For this review, take the finished solid that the model builds, in its own axes (mm). A direction names the side the tool comes from. Give positions to 0.01 mm unless a question says otherwise; leave off trailing zeros. Order: outer loops, then holes, each group sorted by start corner. A loop starts at its lowest first (then second) coordinate and runs counter-clockwise, first axis right, second up.
Item 1: Consider section B-B (z = 12.7). Give the boundary of the cut face in (x, y) (3 decimals), plus the area to 3 significant figures.
Item 2: Consider section D-D (y = 0.5). Give the boundary of the cut face in (x, z) (3 decimals).
Item 3: Consider section A-A (x = 0). Give the boundary of the cut face in (y, z) (3 decimals).
Item 4: Machinability: for faces 4 (the flat face through (5, 5.08, 4)), 5 (the cylindrical face through (7.555, 1.878, 0.992)), 6 (the cylindrical face through (9.52, 3.79, 0.34)), which of the approach directions +Z, -Z, +X, -X, +Y, -Y give a long, thin tool a straight path to every point of the face, cutting with its end or side? Answer none if there is none.
Item 5: Consider section C-C (z = 0). Give the boundary of the cut face in (x, y) (3 decimals).
Item 6: The part is to be moulded in two halves that separate along Z. For faces 1 (the cylindrical face through (-3.6, 4.5, -4.6)), 2 (the flat face through (-8, 2, 0)), 3 (the cylindrical face through (15.87, 1.25, 0.47)), say which applies: released by +Z, released by -Z, zero draft, split by the parting line, or undercut.
Item 7: For probe 1 along X at (y, z) = (4.1, 0) (3 decimals); probe 2 along X at (y, z) = (1.3, -12.7) (3 decimals); probe 3 along Y at (x, z) = (4, 11.5), list the stretches that pass through material, from the lowest coordinate up.
Item 8: For P1, Ø4.5, axis at x = 4, z = -1.5, coming from the -Y side; P2, Ø2, axis at y = 4.5, z = 6.5, coming from the +X side; P3, Ø3, axis at x = 9.5, z = -10, coming from the +Y side, all flat-tipped, find the tip position at first contact; note any pin that passes through.
```python
from build123d import *

# Parameters (mm, degrees)
SKETCH1_R                      = 15.875
BOSS_EXTRUDE1_DEPTH            = 2.54
SKETCH2_R                      = 9.525
BOSS_EXTRUDE2_DEPTH            = 2.54
SKETCH3_R                      = 7.62
CUT_EXTRUDE1_DEPTH             = 3.81
CUT_EXTRUDE2_REACH             = 25.018
SKETCH4_R                      = 5.842
CUT_EXTRUDE3_REACH             = 24.594
SKETCH5_R                      = 1.7
CUT_EXTRUDE5_REACH             = 24.594
CUT_EXTRUDE5_DIRECTION_2_DEPTH = 2.794


with BuildPart() as part:
    # Sketch1 → Boss-Extrude1 (new body)
    with BuildSketch(Plane(origin=(0, 0, 0), x_dir=(1, 0, 0), z_dir=(0, 1, 0))):
        with Locations(Location((0, 0, 0), (0, 0, 270))):
            Circle(SKETCH1_R)
    extrude(amount=BOSS_EXTRUDE1_DEPTH)

    # Sketch2 → Boss-Extrude2 (add)
    with BuildSketch(Plane(origin=(0, 2.54, 0), x_dir=(1, 0, 0), z_dir=(0, 1, 0))):
        with Locations(Location((0, 0, 0), (0, 0, 270))):
            Circle(SKETCH2_R)
    extrude(amount=BOSS_EXTRUDE2_DEPTH)

    # Sketch3 → Cut-Extrude1 (cut)
    with BuildSketch(Plane.XZ):
        with Locations(Location((0, 0, 0), (0, 0, 270))):
            Circle(SKETCH3_R)
    extrude(amount=-CUT_EXTRUDE1_DEPTH, mode=Mode.SUBTRACT)

    # Sketch4 → Cut-Extrude2 (cut, up to next)
    with BuildSketch(Plane(origin=(0, 5.08, 0), x_dir=(1, 0, 0), z_dir=(0, 1, 0)), mode=Mode.PRIVATE) as cut_extrude2_sk1:
        with Locations(Location((0, 0, 0), (0, 0, 270))):
            Circle(SKETCH4_R)
    cut_extrude2_tool1 = extrude(cut_extrude2_sk1.sketch, amount=-CUT_EXTRUDE2_REACH, mode=Mode.PRIVATE) & part.part
    add(cut_extrude2_tool1.solids().sort_by_distance((0, 5.08, 0))[0], mode=Mode.SUBTRACT)

    # Sketch5 → Cut-Extrude3 (cut, up to next)
    with BuildSketch(Plane(origin=(0, 2.54, 0), x_dir=(1, 0, 0), z_dir=(0, 1, 0)), mode=Mode.PRIVATE) as cut_extrude3_sk1:
        with Locations(Location((0, 12.7, 0), (0, 0, 270))):
            Circle(SKETCH5_R)
    cut_extrude3_tool1 = extrude(cut_extrude3_sk1.sketch, amount=-CUT_EXTRUDE3_REACH, mode=Mode.PRIVATE) & part.part
    # Sketch5 → Cut-Extrude3 (cut, up to next)
    with BuildSketch(Plane(origin=(0, 2.54, 0), x_dir=(1, 0, 0), z_dir=(0, 1, 0)), mode=Mode.PRIVATE) as cut_extrude3_sk2:
        with Locations(Location((12.7, 0, 0), (0, 0, 270))):
            Circle(SKETCH5_R)
    cut_extrude3_tool2 = extrude(cut_extrude3_sk2.sketch, amount=-CUT_EXTRUDE3_REACH, mode=Mode.PRIVATE) & part.part
    # Sketch5 → Cut-Extrude3 (cut, up to next)
    with BuildSketch(Plane(origin=(0, 2.54, 0), x_dir=(1, 0, 0), z_dir=(0, 1, 0)), mode=Mode.PRIVATE) as cut_extrude3_sk3:
        with Locations(Location((0, -12.7, 0), (0, 0, 270))):
            Circle(SKETCH5_R)
    cut_extrude3_tool3 = extrude(cut_extrude3_sk3.sketch, amount=-CUT_EXTRUDE3_REACH, mode=Mode.PRIVATE) & part.part
    # Sketch5 → Cut-Extrude3 (cut, up to next)
    with BuildSketch(Plane(origin=(0, 2.54, 0), x_dir=(1, 0, 0), z_dir=(0, 1, 0)), mode=Mode.PRIVATE) as cut_extrude3_sk4:
        with Locations(Location((-12.7, 0, 0), (0, 0, 270))):
            Circle(SKETCH5_R)
    cut_extrude3_tool4 = extrude(cut_extrude3_sk4.sketch, amount=-CUT_EXTRUDE3_REACH, mode=Mode.PRIVATE) & part.part
    add(cut_extrude3_tool1.solids().sort_by_distance((0, 2.54, -12.7))[0], mode=Mode.SUBTRACT)
    add(cut_extrude3_tool2.solids().sort_by_distance((12.7, 2.54, 0))[0], mode=Mode.SUBTRACT)
    add(cut_extrude3_tool3.solids().sort_by_distance((0, 2.54, 12.7))[0], mode=Mode.SUBTRACT)
    add(cut_extrude3_tool4.solids().sort_by_distance((-12.7, 2.54, 0))[0], mode=Mode.SUBTRACT)

    # Sketch6 → Cut-Extrude5 (cut, up to next)
    with BuildSketch(Plane(origin=(0, 2.54, 0), x_dir=(1, 0, 0), z_dir=(0, 1, 0)), mode=Mode.PRIVATE) as cut_extrude5_sk1:
        with BuildLine():
            Line((-8, -13.711878974), (-8, 13.711878974))
            ThreePointArc((-8, 13.711878974), (-15.875, 0), (-8, -13.711878974))
        make_face()
    cut_extrude5_tool1 = extrude(cut_extrude5_sk1.sketch, amount=-CUT_EXTRUDE5_REACH, mode=Mode.PRIVATE) & part.part
    add(cut_extrude5_tool1.solids().sort_by_distance((-11.228338, 2.54, 0))[0], mode=Mode.SUBTRACT)

    # Sketch6 → Cut-Extrude5 direction 2 (cut)
    with BuildSketch(Plane(origin=(0, 2.54, 0), x_dir=(1, 0, 0), z_dir=(0, 1, 0))):
        with BuildLine():
            Line((-8, -13.711878974), (-8, 13.711878974))
            ThreePointArc((-8, 13.711878974), (-15.875, 0), (-8, -13.711878974))
        make_face()
    extrude(amount=CUT_EXTRUDE5_DIRECTION_2_DEPTH, mode=Mode.SUBTRACT)


solid = part.part
```
Resolved:
1. outline: (-8, 0) - (-1.7, 0) - (-1.7, 2.54) - (-8, 2.54) - close; (1.7, 0) - (9.525, 0) - (9.525, 2.54) - (1.7, 2.54) - close
1. area: 35.9 mm2
2. outline: (-8, -13.712) arc R15.875 ccw (long way) to (-8, 13.712) - close; hole circle Ø15.24 at (0, 0); hole circle Ø3.4 at (0, -12.7); hole circle Ø3.4 at (0, 12.7); hole circle Ø3.4 at (12.7, 0)
3. outline: (0, -15.875) - (2.54, -15.875) - (2.54, -14.4) - (0, -14.4) - close; (0, -11) - (2.54, -11) - (2.54, -9.525) - (5.08, -9.525) - (5.08, -5.842) - (3.81, -5.842) - (3.81, -7.62) - (0, -7.62) - close; (0, 7.62) - (3.81, 7.62) - (3.81, 5.842) - (5.08, 5.842) - (5.08, 9.525) - (2.54, 9.525) - (2.54, 11) - (0, 11) - close; (0, 14.4) - (2.54, 14.4) - (2.54, 15.875) - (0, 15.875) - close
4. face 4: +Z, -Z, +X, -X, +Y
4. face 5: -Y
4. face 6: +Y
5. outline: (-8, 0) - (-7.62, 0) - (-7.62, 3.81) - (-5.842, 3.81) - (-5.842, 5.08) - (-8, 5.08) - close; (5.842, 3.81) - (7.62, 3.81) - (7.62, 0) - (11, 0) - (11, 2.54) - (9.525, 2.54) - (9.525, 5.08) - (5.842, 5.08) - close; (14.4, 0) - (15.875, 0) - (15.875, 2.54) - (14.4, 2.54) - close
6. face 1: undercut
6. face 2: zero draft
6. face 3: split by the parting line
7. probe 1: x = -8 to -5.842, 5.842 to 9.525
7. probe 2: x = -8 to -1.7, 1.7 to 9.525
7. probe 3: y = 0 to 2.54
8. P1: stops at y = 3.81
8. P2: stops at x = 7.78
8. P3: stops at y = 2.54
